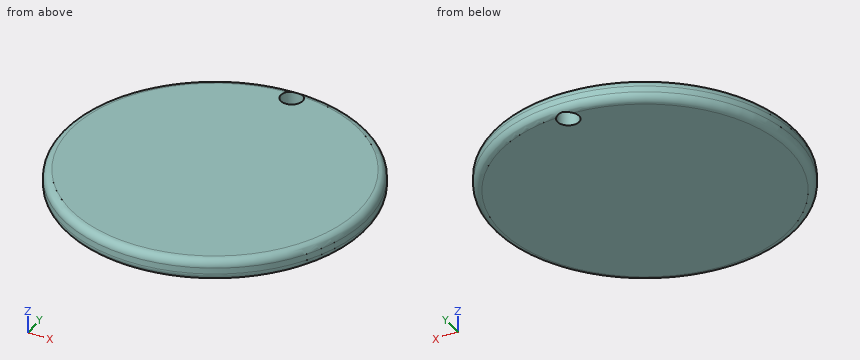
```python
from build123d import *

# Parameters (mm, degrees)
F0_R     = 44.45
F1_DEPTH = 3.175
F2_R     = 3.175
F3_DEPTH = 12.7


# Not quite as in the source:
# - a fillet or chamfer that OpenCascade refuses, or shapes differently, is made with other operations: its cross-section is extruded or revolved along the edge and cut away or added


with BuildPart() as f1:
    # F0 (on Top) → F1 (new body, symmetric)
    with BuildSketch(Plane.XY):
        Circle(F0_R)
    extrude(amount=F1_DEPTH, both=True)

    # F2 (on Top) → F3 (cut, symmetric)
    with BuildSketch(Plane.XY):
        with Locations((0, 40.1277458341)):
            Circle(F2_R)
    extrude(amount=F3_DEPTH, both=True, mode=Mode.SUBTRACT)

    # F4: fillet of radius 2.286 on 2 edges, made by hand

    # F4_s1 → F4_t2 (revolve, cut)
    with BuildSketch(Plane.XZ):
        with BuildLine():
            ThreePointArc((44.45, 0.889), (43.7804461018, 2.5054461018), (42.164, 3.175))
            Line((42.164, 3.175), (44.45, 3.175))
            Line((44.45, 3.175), (44.45, 0.889))
        make_face()
    revolve(axis=Axis((0, 0, 3.175), (0, 0, 1)), mode=Mode.SUBTRACT)

    # F4_s3 → F4_t4 (revolve, cut)
    with BuildSketch(Plane.XZ):
        with BuildLine():
            ThreePointArc((44.45, -0.889), (43.7804461018, -2.5054461018), (42.164, -3.175))
            Line((42.164, -3.175), (44.45, -3.175))
            Line((44.45, -3.175), (44.45, -0.889))
        make_face()
    revolve(axis=Axis((0, 0, -3.175), (0, 0, 1)), mode=Mode.SUBTRACT)


solid = f1.part
```
Check sheet for the modelled part. Datum: model origin and axes. Units: mm. Give positions to 0.01 mm unless a question says otherwise; leave off trailing zeros. Loops run counter-clockwise (first coordinate to the right, second up) from the corner with the lowest first, then second, coordinate; pieces in that order, holes last. Notation, with made-up numbers: M -15,-0.75 L 19,-0.75 A33 cw 19,35.25 Z; hole C 89,77 d2. An arc over 180 degrees is marked long. Answer in a Markdown table with one row per item.
1) Cross-section at A-A (x = 0). Enter the section's corners in (y, z) (3 decimals), plus the area to 3 significant figures.
Solutions:
| item | result |
|---|---|
| outline | M -44.45,-0.889 A2.286 ccw -42.164,-3.175 L 36.953,-3.175 L 36.953,3.175 L -42.164,3.175 A2.286 ccw -44.45,0.889 Z; M 43.303,-2.871 A2.286 ccw 44.45,-0.889 L 44.45,0.889 A2.286 ccw 43.303,2.871 Z |
| area | 520 mm^2 |
2) Depth check by flat-ended pin: pin 1 (10 mm diameter, centred on x = 0, y = 40.13, fed in from -Z) (3 decimals); pin 2 (1 mm diameter, centred on y = 31.5, z = -2, fed in from -X). Enter the tip coordinate at first touch or a pass-through.
Solutions:
| item | result |
|---|---|
| pin 1 | stops at z = -3.175 |
| pin 2 | stops at x = -31.55 |
3) Thickness scan on line 1 (Y direction, x = 0, z = 0.75); line 2 (Y direction, x = 14, z = 0.25); line 3 (Y direction, x = -2.5, z = -2). Record the ranges inside material, lowest first.
Solutions:
| item | result |
|---|---|
| line 1 | y = -44.45 to 36.95, 43.3 to 44.45 |
| line 2 | y = -42.19 to 42.19 |
| line 3 | y = -44.09 to 38.17, 42.08 to 44.09 |
